Geometry: final body of the model. Coordinates: model frame, mm. A direction names the side the tool comes from. Round coordinates to 2 decimals unless told otherwise and drop trailing zeros. Write each loop counter-clockwise with the first axis right and the second up, starting at its lowest first coordinate (ties: lowest second). Pieces come first, ordered by that corner, then holes. Notation, with made-up numbers: M 69.25,54.25 L 94.25,54.25 A10 cw 94.25,65.25 Z; hole C 24,49 d8. An arc over 180 degrees is marked long. Put each result on its own line as item: value. Start each with the question number.
```python
from build123d import *

# Parameters (mm, degrees)
ESBO_O1_R                = 50
RESSALTO_EXTRUS_O2_DEPTH = 5
CORTE_EXTRUS_O3_DEPTH    = 10


with BuildPart() as part:
    # Esboço1 → Ressalto-extrusão2 (new body)
    with BuildSketch(Plane.XY):
        Circle(ESBO_O1_R)
        Polygon((17.205038022, 0), (8.602519011, 14.9), (-8.602519011, 14.9), (-17.205038022, 0), (-8.602519011, -14.9), (8.602519011, -14.9), align=None, mode=Mode.SUBTRACT)
    extrude(amount=RESSALTO_EXTRUS_O2_DEPTH)

    # Esboço2 → Corte-extrusão3 (cut)
    with BuildSketch(Plane.XY.offset(5)):
        with BuildLine():
            ThreePointArc((17.315705324, 28.798343726), (31.728781641, -28.350948037), (-25.332809256, -43.107409748))
            ThreePointArc((-25.332809256, -43.107409748), (24.833037845, -43.397237601), (50, 0))
            ThreePointArc((50, 0), (43.485034201, 24.678974868), (25.637927978, 42.926642647))
            ThreePointArc((25.637927978, 42.926642647), (14.476168491, 39.986199306), (17.315705324, 28.798343726))
        make_face()
        with BuildLine():
            ThreePointArc((25.332809256, 43.107409748), (-43.017296722, 25.485528889), (-25.637927978, -42.926642647))
            ThreePointArc((-25.637927978, -42.926642647), (-14.476168491, -39.986199306), (-17.315705324, -28.798343726))
            ThreePointArc((-17.315705324, -28.798343726), (-31.728781641, 28.350948037), (25.332809256, 43.107409748))
        make_face()
    extrude(amount=-CORTE_EXTRUS_O3_DEPTH, mode=Mode.SUBTRACT)


solid = part.part
```
1) Section A-A, the plane x = 7.5. Output: boundary loops of the cut face in (y, z), and give its area (3 significant figures).
2) First-contact query: pin 1 (1 mm diameter, centred on x = 14.5, y = 37, fed in from -Z); pin 2 (2.5 mm diameter, centred on x = 2.5, z = 3, fed in from -Y); pin 3 (1 mm diameter, centred on x = -19.5, z = 0.5, fed in from +Y). Flat tips, straight axial feed; report the tip coordinate or a pass-through.
3) Ray query, probe 1 along Y at (x, z) = (23, 0.2); probe 2 along X at (y, z) = (6.5, 1.7); probe 3 along Y at (x, z) = (11, 2.7). Return the intervals inside material, ascending.
4) Access query for faces 1 (the face through (12.844, -7.554, 2.465)), 2 (the face through (-17, 1, 5)). Directions: +Z, -Z, +X, -X, +Y, -Y. A direction counts if a zero-diameter tool reaches every point of the face in a straight line with its end or side. Return the directions, or none.
5) Draft query along X for faces 3 (the face through (-17, 1, 0)), 4 (the face through (14.57, 40.14, 2.54)), 5 (the face through (-32.187, 27.558, 2.535)). Return one class per face: +X half, -X half, draft (parallel to the pull), parting line (faces both ways), or undercut.
6) Section C-C, the plane y = 10. Output: boundary loops of the cut face in (x, z).
7) Section D-D, the plane x = 32. Output: boundary loops of the cut face in (y, z), and give its area (3 significant figures).
Solved:
1. outline: M -47.15,0 L -14.9,0 L -14.9,5 L -47.15,5 Z; M 14.9,0 L 48.7,0 L 48.7,5 L 14.9,5 Z
1. area: 330 mm2
2. pin 1: passes through
2. pin 2: stops at y = -48.47
2. pin 3: stops at y = 41.78
3. probe 1: y = -38.75 to 24.69, 43.89 to 44.37
3. probe 2: x = -37.57 to -13.45, 13.45 to 35.33
3. probe 3: y = -45.96 to -10.75, 10.75 to 48.28
4. face 1: +Z, -Z
4. face 2: +Z, +X, -X, +Y, -Y
5. face 3: draft
5. face 4: undercut
5. face 5: parting line
6. outline: M -37.47,0 L -11.43,0 L -11.43,5 L -37.47,5 Z; M 11.43,0 L 33.95,0 L 33.95,5 L 11.43,5 Z
7. outline: M -27.89,0 L 13.83,0 L 13.83,5 L -27.89,5 Z
7. area: 209 mm2
